The listing builds one solid part. Answer for the finished solid, in the listing's coordinates (mm). A direction names the side the tool comes from. Give positions to 0.01 mm unless a question says otherwise; leave off trailing zeros. Order: outer loops, then holes, each group sorted by start corner. A loop starts at its lowest first (then second) coordinate and runs counter-clockwise, first axis right, second up. Notation, with made-up numbers: (74, -38.5) - (122, -38.5) arc R14 cw to (122, -11.5) - close; hole circle Ø8 at (14.25, 49). An arc over 180 degrees is marked (long way). Answer as a JSON object with one key per item and string values. Group by question number.
Q1. A cutting plane is placed at C-C, the plane y = 1.5. Give the vertices of the cut face in (x, z).
Q2. Given pin 1 (1 mm diameter, centred on y = 0.5, z = 42, fed in from -X); pin 2 (3 mm diameter, centred on y = -2, z = 9, fed in from +X); pin 3 (8 mm diameter, centred on x = 14, z = 12.5, fed in from +Y); pin 4 (1 mm diameter, centred on x = 7.5, y = -1, fed in from +Z), each flat-ended and moving along its own axis, determine where each tip first touches the part or whether it passes through.
Q3. A cutting plane is placed at B-B, the plane z = 62. Give the vertices of the cut face in (x, y), and give its area (3 significant figures).
Q4. A cutting plane is placed at D-D, the plane z = 41. Give the vertices of the cut face in (x, y) (1 decimal).
Q5. For faces 4 (the face through (50.8, -1, 13)), 5 (the face through (19, -1.588, 29)), determine the directions among +Z, -Z, +X, -X, +Y, -Y from which every point of the face is accessible in a straight line to the end or side of a thin tool.
Q6. Consider line 1 (Y direction, x = 8, z = 5); line 2 (X direction, y = -2, z = 22); line 3 (X direction, y = -0.25, z = 6.5). Determine where each line is inside the solid, lowest interval first.
Q7. The mould has two halves that part along Y. Classify faces 1 (the face through (-1.58, -0.75, 37.57)), 2 (the face through (0, -1, 76.2)), 3 (the face through (20, 0, 29)): released by +Y, released by -Y, zero draft, split by the parting line, or undercut.
Q8. A cutting plane is placed at A-A, the plane x = 47.5. Give the vertices of the cut face in (y, z).
from build123d import *

# Parameters (mm, degrees)
F1_DEPTH = 76.2
F3_DEPTH = 1.5875


with BuildPart() as f1:
    # F0 (on Top) → F1 (new body)
    with BuildSketch(Plane.XY):
        with BuildLine():
            Line((50.8, 0), (0, 0))
            ThreePointArc((0, 0), (-0.046113, 1.259244), (-0.132987, 2.516333))
            Line((-0.132987, 2.516333), (-1.71473, 2.38125))
            ThreePointArc((-1.71473, 2.38125), (-1.579401, -0.79375), (-1.71473, -3.96875))
            Line((-1.71473, -3.96875), (-0.132987, -4.103833))
            ThreePointArc((-0.132987, -4.103833), (-0.046113, -2.846744), (0, -1.5875))
            Line((0, -1.5875), (50.8, -1.5875))
            Line((50.8, -1.5875), (50.8, 0))
        make_face()
    extrude(amount=F1_DEPTH)

    # F2 (on face) → F3 (cut, through all)
    with BuildSketch(Plane.XZ.offset(1.5875)):
        Polygon((50.8, 76.2), (3.175, 76.2), (50.8, 25.4), align=None)
    extrude(amount=-F3_DEPTH, mode=Mode.SUBTRACT)


solid = f1.part
Reply:
{
 "1": {"outline": "(-1.65, 0) - (-0.06, 0) - (-0.06, 76.2) - (-1.65, 76.2) - close"},
 "2": {"pin 1": "stops at x = -1.62", "pin 2": "stops at x = 50.8", "pin 3": "stops at y = 0", "pin 4": "stops at z = 72.12"},
 "3": {"outline": "(-1.71, -3.97) - (-0.13, -4.1) arc R38.9 ccw to (0, -1.59) - (16.49, -1.59) - (16.49, 0) - (0, 0) arc R38.9 ccw to (-0.13, 2.52) - (-1.71, 2.38) arc R37.31 cw to start", "area": "36.5 mm^2"},
 "4": {"outline": "(-1.7, -4) - (-0.1, -4.1) arc R38.9 ccw to (0, -1.6) - (36.2, -1.6) - (36.2, 0) - (0, 0) arc R38.9 ccw to (-0.1, 2.5) - (-1.7, 2.4) arc R37.3 cw to start"},
 "5": {"face 4": "+Z, -Z, +X, +Y, -Y", "face 5": "+Z, -Z, +X, -Y"},
 "6": {"line 1": "y = -1.59 to 0", "line 2": "x = -1.6 to -0.01", "line 3": "x = -1.58 to 50.8"},
 "7": {"face 1": "undercut", "face 2": "zero draft", "face 3": "released by +Y"},
 "8": {"outline": "(-1.59, 0) - (0, 0) - (0, 28.92) - (-1.59, 28.92) - close"}
}
